Read the model definition and answer for the solid it produces. Units are mm, in the model's axes. A direction names the side the tool comes from. Coordinates: 2 decimals unless noted, no trailing zeros. Write each loop counter-clockwise with the first axis right and the second up, starting at its lowest first coordinate (ties: lowest second). Pieces come first, ordered by that corner, then holes. Notation, with made-up numbers: (69.5, 36) -> (126.5, 36) arc R26 cw to (126.5, 53) -> close; hole circle Ø2 at (56.5, 82.25). An arc over 180 degrees is marked (long way). Answer as a JSON object with one key per item and string values. Group by question number.
(1) Find section D-D (z = -15). Give the vertices of the cut face in (x, y).
(2) Flat-ended cylindrical pins translate along their axes: P1, Ø8.5, axis at x = 60, z = -15, coming from the +Y side; P2, Ø6, axis at x = 51.5, y = 6.5, coming from the -Z side; P3, Ø2, axis at x = 71.5, y = 9, coming from the -Z side; P4, Ø5, axis at y = 5, z = -46.5, coming from the +X side. Find the tip coordinate at first contact, or state that the pin passes through.
(3) Which of the six approach directions +Z, -Z, +X, -X, +Y, -Y give full straight-line access (tool end or side, diameter ignored) to faces 1 (the face through (15, 5, -32)), 2 (the face through (50, 5, -48)), 3 (the face through (25.453, 7.042, -15.716))?
(4) Straight lines are drawn through the part: L1, parallel to X at y = 1.45, z = -15; L2, parallel to X at y = 5.8, z = -15; L3, parallel to Y at x = 43.5, z = -59. For each, find the intervals that lie inside material, in ascending order.
(5) Find section A-A (y = 5). Give the vertices of the cut face in (x, z).
(6) Find section C-C (x = 60). Give the vertices of the cut face in (y, z).
(7) Find section B-B (z = -59). Give the vertices of the cut face in (x, y), then the cut area to 3 significant figures.
(8) For a pull along Z with two mould halves and no side action, classify faces 4 (the face through (0, 5, -18)), 5 (the face through (40, 5, -64)), 6 (the face through (16, 4, -15)) as +Z half, -Z half, draft (parallel to the pull), parting line (faces both ways), or undercut.
from build123d import *

# Parameters (mm, degrees)
EXTRUDE_1_DEPTH     = 10
FILLET_1_R          = 4
SKETCH_2_R          = 2.5
CUT_EXTRUDE_1_DEPTH = 82.829090182
FILLET_2_R          = 4
SKETCH_3_R          = 5.5
CUT_EXTRUDE_2_DEPTH = 6
SKETCH_4_R          = 3.25
CUT_EXTRUDE_3_DEPTH = 103.625532885


with BuildPart() as part:
    # 스케치1 → 보스-돌출1 (new body)
    with BuildSketch(Plane(origin=(0, 0, 0), x_dir=(1, 0, 0), z_dir=(0, 1, 0))):
        Polygon((50, 32), (80, 32), (80, 0), (0, 0), (0, 32), (30, 32), (30, 64), (50, 64), align=None)
    extrude(amount=EXTRUDE_1_DEPTH)

    # 필렛1
    fillet_1_edges = [part.edges().sort_by_distance(p)[0] for p in [
        (40, 10, -64),
        (40, 0, -64),
    ]]
    fillet(fillet_1_edges, radius=FILLET_1_R)

    # 스케치2 → 컷-돌출1 (cut, through all)
    with BuildSketch(Plane(origin=(50, 0, 0), x_dir=(0, 0, -1), z_dir=(1, 0, 0))):
        with Locations((59, 5)):
            Circle(SKETCH_2_R)
    extrude(amount=-CUT_EXTRUDE_1_DEPTH, mode=Mode.SUBTRACT)

    # 필렛2
    fillet_2_edges = [part.edges().sort_by_distance(p)[0] for p in [
        (80, 5, 0),
        (0, 5, 0),
    ]]
    fillet(fillet_2_edges, radius=FILLET_2_R)

    # 스케치3 → 컷-돌출2 (cut)
    with BuildSketch(Plane(origin=(0, 10, 0), x_dir=(1, 0, 0), z_dir=(0, 1, 0))):
        with Locations(Location((20, 15, 0), (0, 0, 270))):
            Circle(SKETCH_3_R)
        with Locations(Location((60, 15, 0), (0, 0, 270))):
            Circle(SKETCH_3_R)
    extrude(amount=-CUT_EXTRUDE_2_DEPTH, mode=Mode.SUBTRACT)

    # 스케치4 → 컷-돌출3 (cut, through all)
    with BuildSketch(Plane(origin=(0, 4, 0), x_dir=(1, 0, 0), z_dir=(0, 1, 0))):
        with Locations(Location((20, 15, 0), (0, 0, 270))):
            Circle(SKETCH_4_R)
        with Locations(Location((60, 15, 0), (0, 0, 270))):
            Circle(SKETCH_4_R)
    extrude(amount=-CUT_EXTRUDE_3_DEPTH, mode=Mode.SUBTRACT)


solid = part.part
Results below:
{
 "1": {"outline": "(0, 0) -> (16.75, 0) -> (16.75, 4) -> (14.5, 4) -> (14.5, 10) -> (0, 10) -> close; (23.25, 0) -> (56.75, 0) -> (56.75, 4) -> (54.5, 4) -> (54.5, 10) -> (25.5, 10) -> (25.5, 4) -> (23.25, 4) -> close; (63.25, 0) -> (80, 0) -> (80, 10) -> (65.5, 10) -> (65.5, 4) -> (63.25, 4) -> close"},
 "2": {"P1": "stops at y = 4", "P2": "stops at z = -64", "P3": "stops at z = -32", "P4": "stops at x = 50"},
 "3": {"face 1": "-Z, -X, +Y, -Y", "face 2": "-Z, +X, +Y, -Y", "face 3": "+Y"},
 "4": {"L1": "x = 0 to 16.75, 23.25 to 56.75, 63.25 to 80", "L2": "x = 0 to 14.5, 25.5 to 54.5, 65.5 to 80", "L3": "y = 0 to 2.5, 7.5 to 10"},
 "5": {"outline": "(0, -32) -> (30, -32) -> (30, -56.5) -> (50, -56.5) -> (50, -32) -> (80, -32) -> (80, -4) arc R4 ccw to (76, 0) -> (4, 0) arc R4 ccw to (0, -4) -> close; (30, -64) -> (50, -64) -> (50, -61.5) -> (30, -61.5) -> close; hole circle Ø11 at (20, -15); hole circle Ø11 at (60, -15)"},
 "6": {"outline": "(0, -32) -> (10, -32) -> (10, -20.5) -> (4, -20.5) -> (4, -18.25) -> (0, -18.25) -> close; (0, -11.75) -> (4, -11.75) -> (4, -9.5) -> (10, -9.5) -> (10, 0) -> (0, 0) -> close"},
 "7": {"outline": "(30, 0) -> (50, 0) -> (50, 2.5) -> (30, 2.5) -> close; (30, 7.5) -> (50, 7.5) -> (50, 10) -> (30, 10) -> close", "area": "100 mm2"},
 "8": {"face 4": "draft", "face 5": "-Z half", "face 6": "undercut"}
}
